Work out the finished part from the listing and answer in its coordinate system (mm). A direction names the side the tool comes from. Give positions to 0.01 mm unless a question says otherwise; leave off trailing zeros. Loops run counter-clockwise (first coordinate to the right, second up) from the corner with the lowest first, then second, coordinate; pieces in that order, holes last. Notation, with made-up numbers: (48, 58) - (103, 58) arc R21 ccw to (103, 97) - close; hole circle Ø8 at (86.5, 3). An arc over 180 degrees is marked (long way). One line per item, written item: value.
from build123d import *

# Parameters (mm, degrees)
F0_W      = 279.4
F0_H      = 25.4
F0_W_2    = 152.4
F0_W_3    = 25.4
F0_W_4    = 127
F1_DEPTH  = 12.7
F2_R      = 3.175
F3_DEPTH  = 50.8
F4_DEPTH  = 25.4
F5_R      = 8.255
F6_DEPTH  = 25.4
F9_R      = 5.8951712564
F10_DEPTH = 25.4


# Not quite as in the source:
# - the program builds the solid bodies; features that only make, move or delete a surface that nothing else refers to are left out


with BuildPart() as f1:
    # F0 (on Front) → F1 (new body, symmetric)
    with BuildSketch(Plane.XZ):
        with Locations((139.7, -12.7)):
            Rectangle(F0_W, F0_H)
        Polygon((0, -25.4), (0, 0), (-25.4, 0), (-25.4, -76.2), (0, -76.2), align=None)
        Polygon((304.8, 0), (279.4, 0), (279.4, -25.4), (279.4, -406.4), (304.8, -406.4), (304.8, -381), (304.8, -228.6), (304.8, -203.2), align=None)
        with Locations((381, -215.9)):
            Rectangle(F0_W_2, F0_H)
        with Locations((381, -393.7)):
            Rectangle(F0_W_2, F0_H)
        Polygon((457.2, 0), (457.2, -203.2), (457.2, -228.6), (457.2, -381), (482.6, -381), (482.6, 0), align=None)
        with Locations((469.9, -393.7)):
            Rectangle(F0_W_3, F0_H)
        with Locations((546.1, -393.7)):
            Rectangle(F0_W_4, F0_H)
        Polygon((609.6, -381), (609.6, -406.4), (635, -406.4), (635, -203.2), (609.6, -203.2), align=None)
    extrude(amount=F1_DEPTH, both=True)

    # F2 (on face) → F3 (cut)
    with BuildSketch(Plane.XZ.offset(12.7)):
        with Locations((469.9, -101.6)):
            Circle(F2_R)
        with Locations((469.9, -50.8)):
            Circle(F2_R)
        with Locations((469.9, -152.4)):
            Circle(F2_R)
        with Locations((469.9, -304.8)):
            Circle(F2_R)
        with Locations((469.9, -254)):
            Circle(F2_R)
        with Locations((469.9, -355.6)):
            Circle(F2_R)
        with Locations((622.3, -304.8)):
            Circle(F2_R)
        with Locations((622.3, -254)):
            Circle(F2_R)
        with Locations((622.3, -355.6)):
            Circle(F2_R)
        with Locations((292.1, -50.8)):
            Circle(F2_R)
    extrude(amount=F3_DEPTH, mode=Mode.SUBTRACT)

    # F2 (on face) → F4 (cut)
    with BuildSketch(Plane.XZ.offset(12.7)):
        with Locations((469.9, -101.6)):
            Circle(F2_R)
        with Locations((469.9, -50.8)):
            Circle(F2_R)
        with Locations((469.9, -152.4)):
            Circle(F2_R)
        with Locations((469.9, -304.8)):
            Circle(F2_R)
        with Locations((469.9, -254)):
            Circle(F2_R)
        with Locations((469.9, -355.6)):
            Circle(F2_R)
        with Locations((622.3, -304.8)):
            Circle(F2_R)
        with Locations((622.3, -254)):
            Circle(F2_R)
        with Locations((622.3, -355.6)):
            Circle(F2_R)
        with Locations((292.1, -50.8)):
            Circle(F2_R)
    extrude(amount=-F4_DEPTH, mode=Mode.SUBTRACT)

    # F5 (on face) → F6 (join)
    with BuildSketch(Plane.XZ.offset(12.7)):
        with Locations((311.5870648182, -30.0990186373)):
            Circle(F5_R)
    extrude(amount=-F6_DEPTH)

    # F9 (on face) → F10 (cut)
    with BuildSketch(Plane.XZ.offset(12.7)):
        with Locations((311.5870648182, -30.0990186373)):
            Circle(F9_R)
    extrude(amount=-F10_DEPTH, mode=Mode.SUBTRACT)


solid = f1.part
1. Find the intervals of material crossed by line 1 along X through (y, z) = (1, -254) (3 decimals); line 2 along X through (y, z) = (0.25, -325); line 3 along X through (y, z) = (-8.75, -30), in increasing order.
Output:
line 1: x = 279.4 to 304.8, 457.2 to 466.725, 473.075 to 482.6, 609.6 to 619.125, 625.475 to 635
line 2: x = 279.4 to 304.8, 457.2 to 482.6, 609.6 to 635
line 3: x = -25.4 to 0, 279.4 to 305.69, 317.48 to 319.84, 457.2 to 482.6
2. Section C-C (z = -87.5) is taken. Write down the section's boundary in (x, y).
Output:
outline: (279.4, -12.7) - (304.8, -12.7) - (304.8, 12.7) - (279.4, 12.7) - close; (457.2, -12.7) - (482.6, -12.7) - (482.6, 12.7) - (457.2, 12.7) - close
3. Section B-B (x = 421) is taken. Write down the section's boundary in (y, z), and give its area (3 significant figures).
Output:
outline: (-12.7, -406.4) - (12.7, -406.4) - (12.7, -381) - (-12.7, -381) - close; (-12.7, -228.6) - (12.7, -228.6) - (12.7, -203.2) - (-12.7, -203.2) - close
area: 1,290 mm²
4. For faces 4 (the flat face through (138, 0, -25.4)), 5 (the flat face through (380, 0, -381)), 6 (the flat face through (545, 0, -381)), determine the directions among +Z, -Z, +X, -X, +Y, -Y from which every point of the face is accessible in a straight line to the end or side of a thin tool.
Output:
face 4: -Z, +Y, -Y
face 5: +Y, -Y
face 6: +Z, +Y, -Y
5. The mould has two halves that part along Z. Classify faces 1 (the flat face through (352, -12.7, -217)), 2 (the flat face through (470, 0, 0)), 3 (the cylindrical face through (319.837, -0.178, -30.392)): released by +Z, released by -Z, zero draft, split by the parting line, or undercut.
Output:
face 1: zero draft
face 2: released by +Z
face 3: undercut
6. Flat-ended cylindrical pins translate along their axes: pin 1 Ø2 at (y, z) = (-2, -183.5) entering from +X; pin 2 Ø5 at (x, z) = (292.1, -50.8) entering from -Y; pin 3 Ø7.5 at (x, y) = (384, 5.5) entering from +Z; pin 4 Ø12 at (y, z) = (4.5, -290) entering from -X. Find the tip coordinate at first contact, or state that the pin passes through.
Output:
pin 1: stops at x = 482.6
pin 2: passes through
pin 3: stops at z = -203.2
pin 4: stops at x = 279.4
7. Section D-D (y = -0.75) is taken. Count the separate pieces of the cut face and the enclosed holes in it, and give its area (3 significant figures).
Output:
separate pieces: 1
enclosed holes: 12
area: 45,600 mm²
8. Section A-A (z = -240) is taken. Write down the section's boundary in (x, y), and give its area (3 significant figures).
Output:
outline: (279.4, -12.7) - (304.8, -12.7) - (304.8, 12.7) - (279.4, 12.7) - close; (457.2, -12.7) - (482.6, -12.7) - (482.6, 12.7) - (457.2, 12.7) - close; (609.6, -12.7) - (635, -12.7) - (635, 12.7) - (609.6, 12.7) - close
area: 1,940 mm²
